```python
from build123d import *

# Parameters (mm, degrees)
F0_W     = 100
F0_H     = 100
F0_R     = 8
F1_DEPTH = 3


with BuildPart() as f1:
    # F0 (on Top) → F1 (new body)
    with BuildSketch(Plane.XY):
        Rectangle(F0_W, F0_H)
        with Locations((-40, -40)):
            Circle(F0_R, mode=Mode.SUBTRACT)
        with Locations((-20, -40)):
            Circle(F0_R, mode=Mode.SUBTRACT)
        with Locations((-40, -20)):
            Circle(F0_R, mode=Mode.SUBTRACT)
        with Locations((-20, -20)):
            Circle(F0_R, mode=Mode.SUBTRACT)
        with Locations((0, -40)):
            Circle(F0_R, mode=Mode.SUBTRACT)
        with Locations((20, -40)):
            Circle(F0_R, mode=Mode.SUBTRACT)
        with Locations((40, -40)):
            Circle(F0_R, mode=Mode.SUBTRACT)
        with Locations((0, -20)):
            Circle(F0_R, mode=Mode.SUBTRACT)
        with Locations((20, -20)):
            Circle(F0_R, mode=Mode.SUBTRACT)
        with Locations((40, -20)):
            Circle(F0_R, mode=Mode.SUBTRACT)
        with Locations((-40, 0)):
            Circle(F0_R, mode=Mode.SUBTRACT)
        with Locations((-40, 20)):
            Circle(F0_R, mode=Mode.SUBTRACT)
        with Locations((-20, 0)):
            Circle(F0_R, mode=Mode.SUBTRACT)
        with Locations((-20, 20)):
            Circle(F0_R, mode=Mode.SUBTRACT)
        with Locations((-40, 40)):
            Circle(F0_R, mode=Mode.SUBTRACT)
        with Locations((-20, 40)):
            Circle(F0_R, mode=Mode.SUBTRACT)
        Circle(F0_R, mode=Mode.SUBTRACT)
        with Locations((20, 0)):
            Circle(F0_R, mode=Mode.SUBTRACT)
        with Locations((0, 20)):
            Circle(F0_R, mode=Mode.SUBTRACT)
        with Locations((20, 20)):
            Circle(F0_R, mode=Mode.SUBTRACT)
        with Locations((40, 0)):
            Circle(F0_R, mode=Mode.SUBTRACT)
        with Locations((40, 20)):
            Circle(F0_R, mode=Mode.SUBTRACT)
        with Locations((0, 40)):
            Circle(F0_R, mode=Mode.SUBTRACT)
        with Locations((20, 40)):
            Circle(F0_R, mode=Mode.SUBTRACT)
        with Locations((40, 40)):
            Circle(F0_R, mode=Mode.SUBTRACT)
    extrude(amount=F1_DEPTH)


solid = f1.part
```
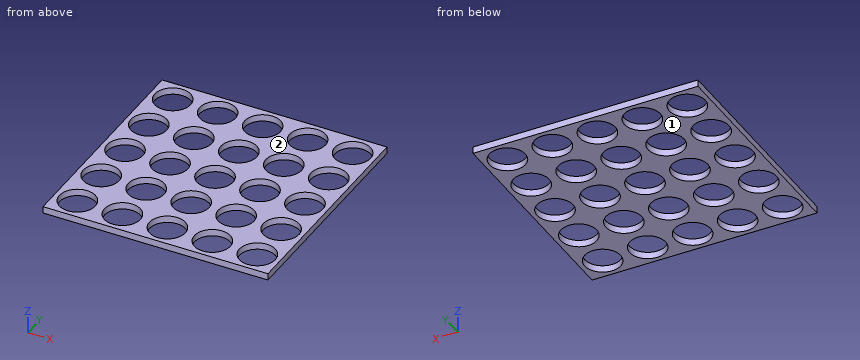
Could you check a few things on this model? Use its own coordinates, in mm. Face numbers are marked on the shaded views. Coordinates: 2 decimals unless noted, no trailing zeros. Order: outer loops, then holes, each group sorted by start corner. A loop starts at its lowest first (then second) coordinate and runs counter-clockwise, first axis right, second up. Notation, with made-up numbers: M 76.25,67 L 116.25,67 A33 cw 116.25,97 Z; hole C 40,12.5 d4. An arc over 180 degrees is marked long. Use one line per item in the form item = value. Start each with the question number.
1. Suppose I cut it at A-A on y = -20. Write out the boundary of the cut face in (x, z), then the cut area to 3 significant figures.
2. Please list where these lines run through material, in increasing order: line 1 (X direction, y = 20.5, z = 2.5); line 2 (Y direction, x = 20, z = 1.7); line 3 (Y direction, x = 3.5, z = 0.4).
3. We'd pull the mould along Z, two halves only. Please class the marked faces 1 and 2: +Z half, -Z half, draft (parallel to the pull), parting line (faces both ways), or undercut.
4. Suppose I cut it at C-C on z = 2.55. Count the separate pieces of the cut face and the enclosed holes in it, then the cut area to 3 significant figures.
5. For pin 1 (9.5 mm diameter, centred on x = 0, y = 0, fed in from +Z), with a flat end and sliding along its axis, tell me the tip position at first contact or that it passes through.
Geometry says:
q1.outline = M -50,0 L -48,0 L -48,3 L -50,3 Z; M -32,0 L -28,0 L -28,3 L -32,3 Z; M -12,0 L -8,0 L -8,3 L -12,3 Z; M 8,0 L 12,0 L 12,3 L 8,3 Z; M 28,0 L 32,0 L 32,3 L 28,3 Z; M 48,0 L 50,0 L 50,3 L 48,3 Z
q1.area = 60.0 mm^2
q2.line_1 = -50 to -47.98, -32.02 to -27.98, -12.02 to -7.98, 7.98 to 12.02, 27.98 to 32.02, 47.98 to 50
q2.line_2 = -50 to -48, -32 to -28, -12 to -8, 8 to 12, 28 to 32, 48 to 50
q2.line_3 = -50 to -47.19, -32.81 to -27.19, -12.81 to -7.19, 7.19 to 12.81, 27.19 to 32.81, 47.19 to 50
q3.face_1 = -Z half
q3.face_2 = +Z half
q4.separate_pieces = 1
q4.enclosed_holes = 25
q4.area = 4,970 mm^2
q5.pin_1 = through
